The model under review builds one solid part; all positions refer to its coordinate system, in mm. Round coordinates to 2 decimals unless told otherwise and drop trailing zeros. Order: outer loops, then holes, each group sorted by start corner. A loop starts at its lowest first (then second) coordinate and runs counter-clockwise, first axis right, second up. Notation, with made-up numbers: (12, -39) - (61, -39) arc R33 cw to (61, 0) - close; hole circle Ø7 at (38, 76). An arc over 180 degrees is marked (long way). One line per question, with ' | ' between items. Start each with the question number.
Item 1: Insertion check: pin 1 Ø5 at (x, y) = (-270, 17) entering from +Z; pin 2 Ø10 at (y, z) = (21, -43.5) entering from +X; pin 3 Ø1.5 at (y, z) = (15.5, -54.5) entering from -X. Each pin has a flat end and moves straight along its axis. Give the tip position at first contact, or say it passes through.
Item 2: Draft analysis for pull direction X (two halves, no side actions). For faces 1 (the face through (-262.6, 8.2, -17)), 2 (the face through (-273.745, 9.328, -49.955)), 3 (the face through (-260.07, 11.63, -49.04)), state which applies: +X half, -X half, draft (parallel to the pull), parting line (faces both ways), or undercut.
Item 3: For L1, parallel to Y at x = -267, z = -39; L2, parallel to Y at x = -268.25, z = -23; L3, parallel to X at y = 8, z = -21, list the stretches that pass through material, from the lowest coordinate up. Write a range as [from, to].
Item 4: Add section C-C on z = -71. State the section outline as (x, y) points, and give its area (3 significant figures).
Item 5: Add section A-A on x = -267. State the section outline as (y, z) points.
Item 6: Add section B-B on y = 14.5. State the section outline as (x, z) points.
from build123d import *

# Parameters (mm, degrees)
SKETCH020_R     = 8.5
PAD013_DEPTH    = 65
SKETCH022_R     = 7.5
POCKET001_DEPTH = 85
SKETCH_R        = 7
POCKET_DEPTH    = 70


with BuildPart() as part:
    # Sketch020 → Pad013 (new body)
    with BuildSketch(Plane.XY):
        Circle(SKETCH020_R)
    extrude(amount=PAD013_DEPTH)

    # Sketch022 (on Face3 of Pad013) → Pocket001 (cut)
    with BuildSketch(Plane.XY.offset(65)):
        Circle(SKETCH022_R)
    extrude(amount=-POCKET001_DEPTH, mode=Mode.SUBTRACT)

    # Sketch (on Face3 of Pad013) → Pocket (cut)
    with BuildSketch(Plane.XY.offset(65)):
        Circle(SKETCH_R)
    extrude(amount=-POCKET_DEPTH, mode=Mode.SUBTRACT)


with BuildPart() as part_1:
    # Body009 placement: moved
    add(part.part.moved(Location((-267, 14.5, -82))))


solid = part_1.part
Determined:
1) pin 1: through | pin 2: x = -258.63 | pin 3: x = -275.5
2) face 1: draft | face 2: parting line | face 3: undercut
3) L1: [6, 7], [22, 23] | L2: [6.09, 7.1], [21.9, 22.91] | L3: [-272.48, -270.74], [-263.26, -261.52]
4) outline: circle Ø17 at (-267, 14.5); hole circle Ø15 at (-267, 14.5) | area: 50.3 mm2
5) outline: (6, -82) - (7, -82) - (7, -17) - (6, -17) - close; (22, -82) - (23, -82) - (23, -17) - (22, -17) - close
6) outline: (-275.5, -82) - (-274.5, -82) - (-274.5, -17) - (-275.5, -17) - close; (-259.5, -82) - (-258.5, -82) - (-258.5, -17) - (-259.5, -17) - close
